Geometry check sheet. Reference: drawing and pictorial views, mm from the part's lowest x, y, z. Give positions to 0.01 mm unless a question says otherwise; leave off trailing zeros. Write each loop counter-clockwise with the first axis right and the second up, starting at its lowest first coordinate (ties: lowest second). Pieces come first, ordered by that corner, then holes. Notation, with made-up numbers: M 3.5,-3.75 L 9.5,-3.75 A8 cw 9.5,4.25 Z; hole C 68.25,2.5 d9. An arc over 180 degrees is marked long. Write item = value, one per line. Start each with the question number.
1) Mould release check, pull along Y, two halves, no side actions. Record for the marked faces 1, 2 and 3: released by +Y, released by -Y, zero draft, split by the parting line, or undercut.
2) Scan lines: line 1 along Y through (x, z) = (1.75, 16); line 2 along X through (y, z) = (11.5, 12.75); line 3 along X through (y, z) = (14.5, 8.5). Record each from-to range of solid material in increasing order. Write a range as [from, to].
3) Go/stop test with flat-tipped pins: pin 1 (1 mm diameter, centred on x = 4.5, y = 61.5, fed in from +Z); pin 2 (1 mm diameter, centred on y = 50, z = 7, fed in from -X); pin 3 (1.5 mm diameter, centred on x = 12.5, y = 46.5, fed in from +Z). Record where each tip stops, or that it passes through.
4) Cross-section at C-C, the plane y = 9. Record the cut outline in (x, z).
5) Cross-section at B-B, the plane x = 12.5. Record the cut outline in (y, z), plus the area to 3 significant figures.
6) Cross-section at A-A, the plane z = 12.5. Record the cut outline in (x, y), plus the area to 3 significant figures.
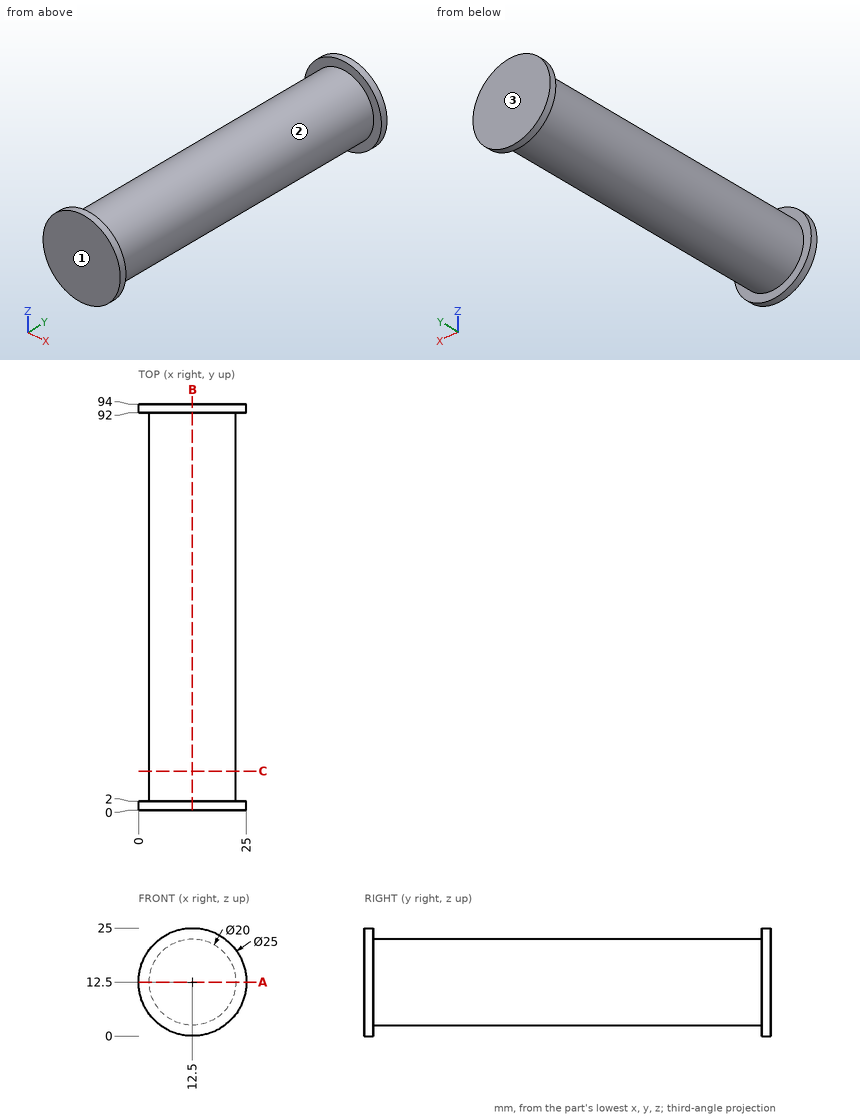
Reply:
q1.face_1 = released by -Y
q1.face_2 = undercut
q1.face_3 = released by +Y
q2.line_1 = [0, 2], [92, 94]
q2.line_2 = [2.5, 22.5]
q2.line_3 = [3.33, 21.67]
q3.pin_1 = 19.11
q3.pin_2 = 3.84
q3.pin_3 = 22.5
q4.outline = C 12.5,12.5 d20
q5.outline = M 0,0 L 2,0 L 2,2.5 L 92,2.5 L 92,0 L 94,0 L 94,25 L 92,25 L 92,22.5 L 2,22.5 L 2,25 L 0,25 Z
q5.area = 1,900 mm2
q6.outline = M 0,0 L 25,0 L 25,2 L 22.5,2 L 22.5,92 L 25,92 L 25,94 L 0,94 L 0,92 L 2.5,92 L 2.5,2 L 0,2 Z
q6.area = 1,900 mm2
